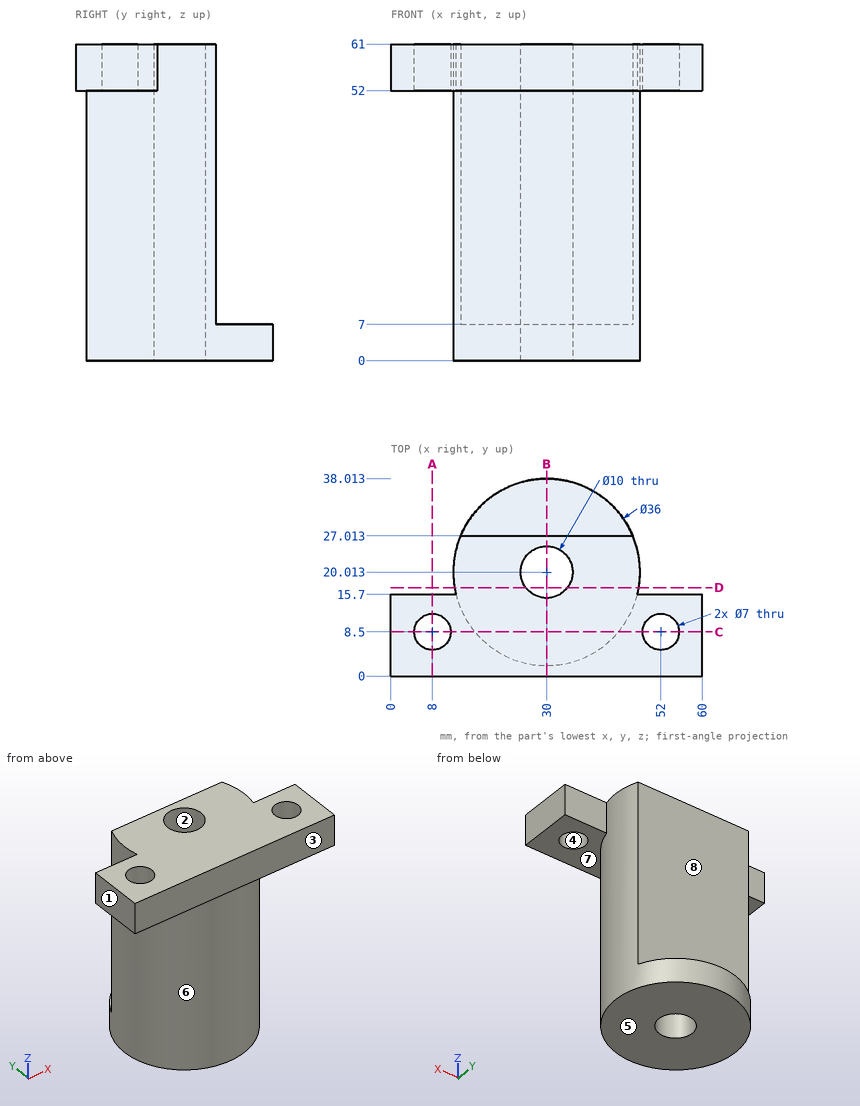
Design review of the part shown in the three views and the two pictorial views. Dimensions are in mm from the part's minimum x, y and z. A direction names the side the tool comes from. Give positions to 0.01 mm unless a question says otherwise; leave off trailing zeros. Order: outer loops, then holes, each group sorted by start corner. A loop starts at its lowest first (then second) coordinate and runs counter-clockwise, first axis right, second up. Notation, with made-up numbers: M 23.25,31 L 46.25,31 A17 cw 46.25,54 Z; hole C -16.5,22 d6. An arc over 180 degrees is marked long. Answer in a Markdown table with one row per item. Add a question column.
(1) Consider section A-A on x = 8. State the section outline as (y, z) points.
(2) For pin 1 (6 mm diameter, centred on x = 39.5, z = 31.5, fed in from +Y); pin 2 (4.5 mm diameter, centred on x = 55.5, z = 55, fed in from +Y); pin 3 (9 mm diameter, centred on x = 37.5, y = 33.5, fed in from +Z), all flat-tipped, find the tip position at first contact; note any pin that passes through.
(3) Consider section C-C on y = 8.5. State the section outline as (x, z) points, and give its area (3 significant figures).
(4) Consider section D-D on y = 17. State the section outline as (x, z) points, and give its area (3 significant figures).
(5) For the marked faces 5, 6, 7 and 8, list the 3-axis set-ups (+Z, -Z, +X, -X, +Y, -Y) from which the entire face can be reached by the end or side of a thin tool; tool diameter is ignored.
(6) Mouldability with a two-part tool opening along X and no side actions: class the marked faces 1, 2, 3 and 4 as +X half, -X half, draft (parallel to the pull), parting line (faces both ways), or undercut.
(7) Consider section B-B on x = 30. State the section outline as (y, z) points.
(8) Wall thickness on probe 1 along Y at (x, z) = (30, 30.5); probe 2 along Y at (x, z) = (8, 57.75); probe 3 along Z at (x, y) = (57, 13): over which ranges is each line inside the solid? List them lowest first. Write a range as [from, to].
Evaluation:
| question | item | result |
|---|---|---|
| 1 | outline | M 0,52 L 5,52 L 5,61 L 0,61 Z; M 12,52 L 15.7,52 L 15.7,61 L 12,61 Z |
| 2 | pin 1 | stops at y = 27.01 |
| 2 | pin 2 | stops at y = 15.7 |
| 2 | pin 3 | stops at z = 7 |
| 3 | outline | M 0,52 L 4.5,52 L 4.5,61 L 0,61 Z; M 11.5,52 L 16.16,52 L 16.16,0 L 43.84,0 L 43.84,52 L 48.5,52 L 48.5,61 L 11.5,61 Z; M 55.5,52 L 60,52 L 60,61 L 55.5,61 Z |
| 3 | area | 1,850 mm^2 |
| 4 | outline | M 12.25,0 L 26.01,0 L 26.01,61 L 12.25,61 Z; M 33.99,0 L 47.75,0 L 47.75,61 L 33.99,61 Z |
| 4 | area | 1,680 mm^2 |
| 5 | face 5 | -Z, +X, -X, +Y, -Y |
| 5 | face 6 | -Z |
| 5 | face 7 | -Z, -Y |
| 5 | face 8 | +Z, +X, -X, +Y |
| 6 | face 1 | -X half |
| 6 | face 2 | undercut |
| 6 | face 3 | draft |
| 6 | face 4 | undercut |
| 7 | outline | M 0,52 L 2.01,52 L 2.01,0 L 15.01,0 L 15.01,61 L 0,61 Z; M 25.01,0 L 38.01,0 L 38.01,7 L 27.01,7 L 27.01,61 L 25.01,61 Z |
| 8 | probe 1 | y = [2.01, 15.01], [25.01, 27.01] |
| 8 | probe 2 | y = [0, 5], [12, 15.7] |
| 8 | probe 3 | z = [52, 61] |
